CAD build for the part. Positions are in the model's coordinates, mm. Face numbers are marked on the shaded views. A direction names the side the tool comes from. Coordinates: 2 decimals unless noted, no trailing zeros. Write each loop counter-clockwise with the first axis right and the second up, starting at its lowest first coordinate (ties: lowest second). Pieces come first, ordered by that corner, then holes. Notation, with made-up numbers: (42.5, -31) - (77.5, -31) arc R13 ccw to (77.5, -22) - close; hole circle Ø8 at (0.25, 48). An arc over 180 degrees is marked (long way). One line per question, with ' | ' between items. Start each with the question number.
1. Flat gauge pins, fed straight in: P1, Ø13.5, axis at y = 21, z = 19, coming from the +X side; P2, Ø11, axis at y = 2, z = -19, coming from the +X side; P3, Ø3, axis at x = -41, z = -85.5, coming from the -Y side. Where does each tip first touch, or does it go through?
2. Which spindle directions (+Z, -Z, +X, -X, +Y, -Y) get a long thin tool onto all of the face, cutting with end or side? Do the marked faces 1, 2, 3 and 4. Say none if no direction does.
3. Probe line 1 (X direction, y = 28.5, z = -18.5); line 2 (Y direction, x = 2, z = -48.5); line 3 (Y direction, x = -1, z = -63). List the from-to ranges inside material, lowest first.
4. Band-saw the part on D-D, the plane x = 17. Write the cut outline in (y, z).
5. Two-plate mould, pull along Y, no slides. Class the marked faces 5, 6 and 7: +Y half, -Y half, draft (parallel to the pull), parting line (faces both ways), or undercut.
6. Band-saw the part on C-C, the plane y = 57. Write the cut outline in (x, z), then the cut area to 3 significant figures.
7. Band-saw the part on B-B, the plane x = 0. Write the cut outline in (y, z), then the cut area to 4 significant figures.
8. Band-saw the part on A-A, the plane z = 57.5. Write the cut outline in (x, y), then the cut area to 3 significant figures.
from build123d import *

# Parameters (mm, degrees)
SKETCH1_R                = 6
BOSS_EXTRUDE1_DEPTH      = 5
SKETCH2_W                = 75
SKETCH2_H                = 100
BOSS_EXTRUDE2_DEPTH      = 30
BOSS_EXTRUDE3_DEPTH      = 60
BOSS_EXTRUDE3_DEPTH_BACK = 160
SKETCH3_R                = 75


with BuildPart() as part:
    # Sketch1 → Boss-Extrude1 (new, symmetric)
    with BuildSketch(Plane(origin=(0, 0, 0), x_dir=(1, 0, 0), z_dir=(0, 1, 0))):
        with BuildLine():
            Line((-47, 80), (47, 80))
            ThreePointArc((47, 80), (60.656854249, 85.656854249), (55, 72))
            Line((55, 72), (55, -72))
            ThreePointArc((55, -72), (60.656854249, -85.656854249), (47, -80))
            Line((47, -80), (-47, -80))
            ThreePointArc((-47, -80), (-60.656854249, -85.656854249), (-55, -72))
            Line((-55, -72), (-55, 72))
            ThreePointArc((-55, 72), (-60.656854249, 85.656854249), (-47, 80))
        make_face()
        with Locations(Location((55, 80, 0), (0, 0, 270))):
            Circle(SKETCH1_R, mode=Mode.SUBTRACT)
        with Locations(Location((-55, 80, 0), (0, 0, 270))):
            Circle(SKETCH1_R, mode=Mode.SUBTRACT)
        with Locations(Location((55, -80, 0), (0, 0, 90))):
            Circle(SKETCH1_R, mode=Mode.SUBTRACT)
        with Locations(Location((-55, -80, 0), (0, 0, 90))):
            Circle(SKETCH1_R, mode=Mode.SUBTRACT)
    extrude(amount=BOSS_EXTRUDE1_DEPTH, both=True)

    # Sketch2 → Boss-Extrude2 (add)
    with BuildSketch(Plane(origin=(0, 5, 0), x_dir=(1, 0, 0), z_dir=(0, 1, 0))):
        Rectangle(SKETCH2_W, SKETCH2_H)
    extrude(amount=BOSS_EXTRUDE2_DEPTH)

    # Sketch3 → Boss-Extrude3 (add, two sides: drawn at the far end of the back side and taken through both)
    with BuildSketch(Plane.XY.offset(50).offset(-BOSS_EXTRUDE3_DEPTH_BACK)):
        with Locations((0, 96.5)):
            Circle(SKETCH3_R)
    extrude(amount=BOSS_EXTRUDE3_DEPTH + BOSS_EXTRUDE3_DEPTH_BACK)


solid = part.part
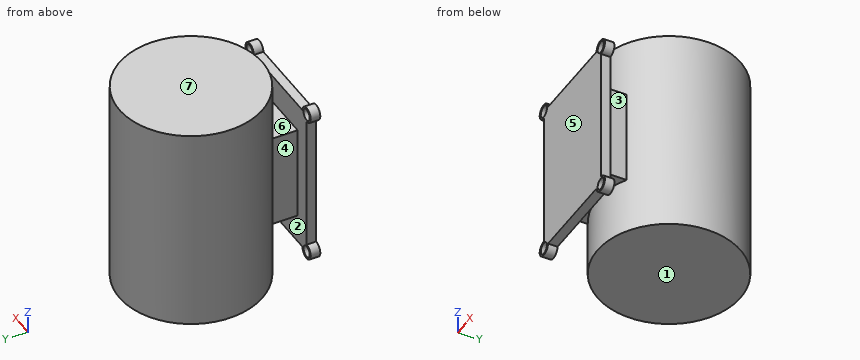
Filled in:
1) P1: stops at x = 37.5 | P2: stops at x = 55 | P3: stops at y = 32.74
2) face 1: -Z, +X, -X, +Y, -Y | face 2: none | face 3: +Z, -Z, +X | face 4: +Z, -Z, -X
3) line 1: x = -37.5 to 37.5 | line 2: y = -5 to 171.47 | line 3: y = -5 to 5, 21.51 to 171.49
4) outline: (-5, -80) - (5, -80) - (5, -50) - (23.45, -50) - (23.45, -110) - (169.55, -110) - (169.55, 110) - (23.45, 110) - (23.45, 50) - (5, 50) - (5, 80) - (-5, 80) - close
5) face 5: -Y half | face 6: undercut | face 7: draft
6) outline: (-63.76, -110) - (63.76, -110) - (63.76, 110) - (-63.76, 110) - close | area: 28,100 mm²
7) outline: (-5, -80) - (5, -80) - (5, -50) - (21.5, -50) - (21.5, -110) - (171.5, -110) - (171.5, 110) - (21.5, 110) - (21.5, 50) - (5, 50) - (5, 80) - (-5, 80) - close | area: 36,250 mm²
8) outline: circle Ø150 at (0, 96.5); (-55, -5) - (55, -5) - (55, 5) - (-55, 5) - close | area: 18,800 mm²
